from build123d import *

# Parameters (mm, degrees)
F1_DEPTH       = 44.45
F3_D           = 6.35
F3_CSINK_D     = 10.16
F3_CSINK_ANGLE = 82
F4_T1_DEPTH    = 68.1485226281
F5_R           = 1.27


# Not quite as in the source:
# - a fillet or chamfer that OpenCascade refuses, or shapes differently, is made with other operations: its cross-section is extruded or revolved along the edge and cut away or added
# - a feature names something its author has since deleted; it is built from what else it names


with BuildPart() as f1:
    # F0 (on Top) → F1 (new body)
    with BuildSketch(Plane.XY):
        Polygon((0, 83.7955678842), (0, 0), (19.05, 0), (19.05, 50.8), align=None)
    extrude(amount=F1_DEPTH)

    # F3 (through all)
    with Locations(Plane(origin=(0, 0, 0), x_dir=(0, -1, 0), z_dir=(-1, 0, 0))):
        with Locations((-12.7, 22.225), (-38.1, 22.225)):
            CounterSinkHole(F3_D / 2, F3_CSINK_D / 2, counter_sink_angle=F3_CSINK_ANGLE)

    # F4: fillet of radius 1.27 on 1 edges, made by hand

    # F4_s2 → F4_t1 (cut)
    with BuildSketch(Plane.XY.offset(-11.849261314)):
        with BuildLine():
            ThreePointArc((0, 79.0558633586), (0.9412998127, 80.282589158), (2.3698522628, 79.6908633586))
            Line((2.3698522628, 79.6908633586), (0, 83.7955678842))
            Line((0, 83.7955678842), (0, 79.0558633586))
        make_face()
    extrude(amount=F4_T1_DEPTH, mode=Mode.SUBTRACT)

    # F5
    f5_edges = [f1.edges().sort_by_distance(p)[0] for p in [
        (0.9413, 80.282589, 44.45),
        (10.709926, 65.245432, 44.45),
        (19.05, 25.4, 44.45),
        (9.525, 0, 44.45),
        (0, 39.527932, 44.45),
        (0.9413, 80.282589, 0),
        (10.709926, 65.245432, 0),
        (19.05, 25.4, 0),
        (9.525, 0, 0),
        (0, 39.527932, 0),
        (0, 0, 22.225),
        (19.05, 0, 22.225),
    ]]
    fillet(f5_edges, radius=F5_R)


solid = f1.part
Geometry: final body of the model. Coordinates: model frame, mm. Round coordinates to 2 decimals unless told otherwise and drop trailing zeros. Loops run counter-clockwise (first coordinate to the right, second up) from the corner with the lowest first, then second, coordinate; pieces in that order, holes last. Notation, with made-up numbers: (37.5, -15.75) -> (89.5, -15.75) arc R27 ccw to (89.5, 14.25) -> close; hole circle Ø1 at (69.5, -3.75). An arc over 180 degrees is marked (long way). One line per question, with ' | ' between items. Start each with the question number.
1. Section C-C on x = 5.5. Count the separate pieces of the cut face and the enclosed holes in it, and give its area (3 significant figures).
2. Section A-A on y = 12.7. Output: boundary loops of the cut face in (x, z) (3 decimals), and give its area (3 significant figures).
3. Mould query, pull axis Z, two halves, no side actions, for faces 1 (the face through (0.919, 80.276, 21.932)), 2 (the face through (9, 32, 0)), 3 (the face through (10.74, 10.36, 24.37)). Classes: pulls with the +Z half, pulls with the -Z half, needs draft (parallel to the pull), parting line crosses it, or undercut.
4. Contact query for flat-ended pins moving along their axis: pin 1 (8.5 mm diameter, centred on y = 38.1, z = 22.225, fed in from -X); pin 2 (6 mm diameter, centred on x = 11.5, z = 21, fed in from +Y). Output: stop coordinate, or through.
5. Section B-B on z = 9.5. Output: boundary loops of the cut face in (x, y), and give its area (3 significant figures).
6. Line query: line 1 along Z through (x, y) = (15, 38.1); line 2 along Y through (x, z) = (14.5, 21); line 3 along Y through (x, z) = (7.25, 22.5). Output: solid intervals per line, ascending. Write a range as [from, to].
Returned:
1) separate pieces: 1 | enclosed holes: 2 | area: 3,240 mm2
2) outline: (0, 1.27) arc R1.27 ccw to (1.27, 0) -> (17.78, 0) arc R1.27 ccw to (19.05, 1.27) -> (19.05, 19.05) -> (2.191, 19.05) -> (0, 17.145) -> close; (0, 27.305) -> (2.191, 25.4) -> (19.05, 25.4) -> (19.05, 43.18) arc R1.27 ccw to (17.78, 44.45) -> (1.27, 44.45) arc R1.27 ccw to (0, 43.18) -> close | area: 720 mm2
3) face 1: needs draft | face 2: pulls with the -Z half | face 3: undercut
4) pin 1: stops at x = 0.95 | pin 2: stops at y = 69.07
5) outline: (0, 1.27) arc R1.27 ccw to (1.27, 0) -> (17.78, 0) arc R1.27 ccw to (19.05, 1.27) -> (19.05, 50.8) -> (2.37, 79.69) arc R1.27 ccw to (0, 79.06) -> close | area: 1,280 mm2
6) line 1: z = [0, 19.05], [25.4, 44.45] | line 2: y = [0, 9.77], [15.63, 35.17], [41.03, 58.68] | line 3: y = [0, 9.54], [15.86, 34.94], [41.26, 71.24]
